Could you check a few things on this model? Use its own coordinates, in mm. Face numbers are marked on the shaded views. A direction names the side the tool comes from. Coordinates: 2 decimals unless noted, no trailing zeros. Order: outer loops, then holes, each group sorted by start corner. A loop starts at its lowest first (then second) coordinate and runs counter-clockwise, first axis right, second up. Notation, with made-up numbers: (-26, 70) - (5, 70) arc R29 cw to (5, 95) - close; hole circle Ø5 at (82.25, 38.5). An arc over 180 degrees is marked (long way). Answer as a JSON object with one key per item and string values. Group by question number.
(1) Imagine slicing it at B-B, the plane z = -50. Write out the boundary of the cut face in (x, y).
(2) Imagine slicing it at A-A, the plane y = 37. Write out the boundary of the cut face in (x, z).
(3) Please list where these lines run through material, in increasing order: probe 1 along Y at (x, z) = (84, -105); probe 2 along X at (y, z) = (48, -58.5); probe 3 along X at (y, z) = (25, -136) (3 decimals).
(4) We'd pull the mould along X, two halves only. Please class the marked faces 4, 5 and 6: pulls with the +X half, pulls with the -X half, needs draft (parallel to the pull), parting line crosses it, or undercut.
(5) Will these pins go through, and if not, where does the flat tip stop? P1, Ø11.5, axis at y = 20.425, z = -105, coming from the +X side (3 decimals); P2, Ø6, axis at x = 162, y = 21, coming from the -Z side; P3, Ø3, axis at y = 28.5, z = -70, coming from the -X side.
(6) Which directions (+Z, -Z, +X, -X, +Y, -Y) give clear straight access to the entire face, cutting with the end or side of a thin tool? Please do the marked faces 1, 2 and 3.
(7) Imagine slicing it at C-C, the plane y = 56. Write out the boundary of the cut face in (x, z).
(8) Imagine slicing it at D-D, the plane x = 184.5. Write out the boundary of the cut face in (y, z), and give its area (3 significant figures).
from build123d import *

# Parameters (mm, degrees)
SKETCH1_W           = 245
SKETCH1_H           = 160
BOSS_EXTRUDE1_DEPTH = 10
SKETCH2_W           = 15
SKETCH2_H           = 40
BOSS_EXTRUDE3_DEPTH = 60
SKETCH3_R           = 5
CUT_EXTRUDE1_DEPTH  = 146
CHAMFER1_SIZE       = 10
CHAMFER2_SIZE       = 3
FILLET1_R           = 1
SKETCH4_W           = 10
SKETCH4_H           = 60
BOSS_EXTRUDE4_DEPTH = 20.85
SKETCH7_R           = 5.075
CUT_EXTRUDE2_DEPTH  = 86
FILLET2_R           = 1


with BuildPart() as part:
    # Sketch1 → Boss-Extrude1 (new body)
    with BuildSketch(Plane(origin=(0, 0, 0), x_dir=(1, 0, 0), z_dir=(0, 1, 0))):
        with Locations((122.5, 80)):
            Rectangle(SKETCH1_W, SKETCH1_H)
    extrude(amount=BOSS_EXTRUDE1_DEPTH)

    # Sketch2 → Boss-Extrude3 (add)
    with BuildSketch(Plane(origin=(0, 10, 0), x_dir=(1, 0, 0), z_dir=(0, 1, 0))):
        with Locations((57.5, 50)):
            Rectangle(SKETCH2_W, SKETCH2_H)
        with Locations((187.5, 50)):
            Rectangle(SKETCH2_W, SKETCH2_H)
    extrude(amount=BOSS_EXTRUDE3_DEPTH)

    # Sketch3 → Cut-Extrude1 (cut)
    with BuildSketch(Plane(origin=(195, 0, 0), x_dir=(0, 0, -1), z_dir=(1, 0, 0))):
        with Locations((50, 56)):
            Circle(SKETCH3_R)
    extrude(amount=-CUT_EXTRUDE1_DEPTH, mode=Mode.SUBTRACT)

    # Chamfer1
    chamfer1_edges = [part.edges().sort_by_distance(p)[0] for p in [
        (65, 10, -50),
        (57.5, 10, -70),
        (50, 10, -50),
        (57.5, 10, -30),
        (195, 10, -50),
        (187.5, 10, -70),
        (180, 10, -50),
        (187.5, 10, -30),
    ]]
    chamfer(chamfer1_edges, length=CHAMFER1_SIZE)

    # Chamfer2
    chamfer2_edges = [part.edges().sort_by_distance(p)[0] for p in [
        (57.5, 70, -70),
        (57.5, 70, -30),
        (187.5, 70, -70),
        (187.5, 70, -30),
    ]]
    chamfer(chamfer2_edges, length=CHAMFER2_SIZE)

    # Fillet1
    fillet1_edges = [part.edges().sort_by_distance(p)[0] for p in [
        (57.5, 70, -67),
        (57.5, 70, -33),
        (57.5, 67, -30),
        (57.5, 67, -70),
        (187.5, 70, -33),
        (187.5, 70, -67),
        (187.5, 67, -70),
        (187.5, 67, -30),
    ]]
    fillet(fillet1_edges, radius=FILLET1_R)

    # Sketch4 → Boss-Extrude4 (add)
    with BuildSketch(Plane(origin=(0, 10, 0), x_dir=(1, 0, 0), z_dir=(0, 1, 0))):
        with Locations((85.625, 125)):
            Rectangle(SKETCH4_W, SKETCH4_H)
        with Locations((159.375, 125)):
            Rectangle(SKETCH4_W, SKETCH4_H)
    extrude(amount=BOSS_EXTRUDE4_DEPTH)

    # Sketch7 → Cut-Extrude2 (cut)
    with BuildSketch(Plane(origin=(164.375, 0, 0), x_dir=(0, 0, -1), z_dir=(1, 0, 0))):
        with Locations((105, 20.425)):
            Circle(SKETCH7_R)
        with Locations((145, 20.425)):
            Circle(SKETCH7_R)
    extrude(amount=-CUT_EXTRUDE2_DEPTH, mode=Mode.SUBTRACT)

    # Fillet2
    fillet2_edges = [part.edges().sort_by_distance(p)[0] for p in [
        (90.625, 10, -125),
        (80.625, 10, -125),
        (164.375, 10, -125),
        (154.375, 10, -125),
    ]]
    fillet(fillet2_edges, radius=FILLET2_R)


solid = part.part
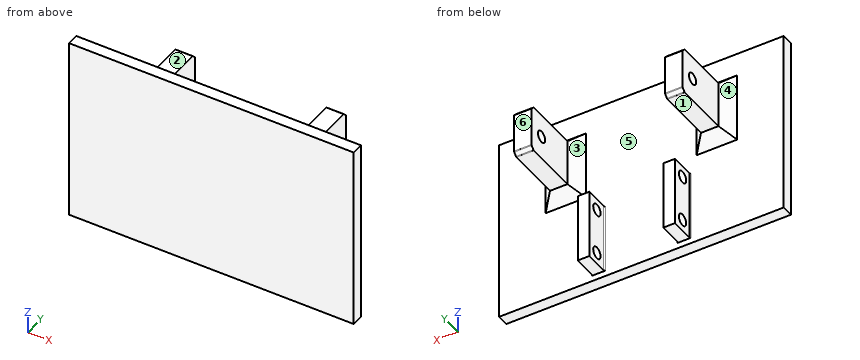
Result set:
{
 "1": {"outline": "(0, 0) - (245, 0) - (245, 10) - (205, 10) - (195, 20) - (195, 51) - (180, 51) - (180, 20) - (170, 10) - (75, 10) - (65, 20) - (65, 51) - (50, 51) - (50, 20) - (40, 10) - (0, 10) - close; (50, 61) - (65, 61) - (65, 70) - (50, 70) - close; (180, 61) - (195, 61) - (195, 70) - (180, 70) - close"},
 "2": {"outline": "(50, -70) - (65, -70) - (65, -30) - (50, -30) - close; (180, -70) - (195, -70) - (195, -30) - (180, -30) - close"},
 "3": {"probe 1": "y = 0 to 15.35, 25.5 to 30.85", "probe 2": "x = 50 to 65, 180 to 195", "probe 3": "x = 80.625 to 90.625, 154.375 to 164.375"},
 "4": {"face 4": "pulls with the -X half", "face 5": "undercut", "face 6": "needs draft"},
 "5": {"P1": "stops at x = 164.375", "P2": "stops at z = -155", "P3": "stops at x = 50"},
 "6": {"face 1": "-Z, +X, -X, +Y", "face 2": "+Z, +X, -X, +Y", "face 3": "+Z, -Z, +Y"},
 "7": {"outline": "(50, -70) - (65, -70) - (65, -55) - (50, -55) - close; (50, -45) - (65, -45) - (65, -30) - (50, -30) - close; (180, -70) - (195, -70) - (195, -55) - (180, -55) - close; (180, -45) - (195, -45) - (195, -30) - (180, -30) - close"},
 "8": {"outline": "(0, -160) - (10, -160) - (10, -80) - (20, -70) - (66.59, -70) arc R1 ccw to (67.29, -69.71) - (69.71, -67.29) arc R1 ccw to (70, -66.59) - (70, -33.41) arc R1 ccw to (69.71, -32.71) - (67.29, -30.29) arc R1 ccw to (66.59, -30) - (20, -30) - (10, -20) - (10, 0) - (0, 0) - close; hole circle Ø10 at (56, -50)", "area": "4,010 mm^2"}
}
